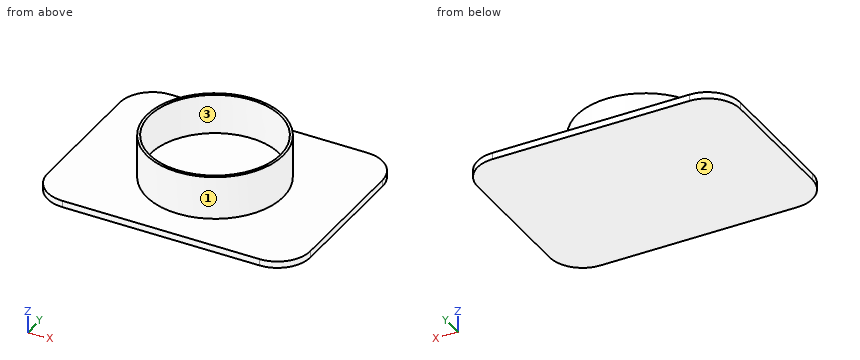
```python
from build123d import *

# Parameters (mm, degrees)
ESQUISSE1_R             = 10.4
BOSS_EXTRU_1_DEPTH      = 6.6
ESQUISSE2_R             = 10
ENL_V_MAT_EXTRU_1_DEPTH = 6
ENL_V_MAT_EXTRU_1_TAPER = 1
ESQUISSE3_W             = 40
ESQUISSE3_H             = 30
BOSS_EXTRU_2_DEPTH      = 1
CONG_1_R                = 5


with BuildPart() as part:
    # Esquisse1 → Boss.-Extru.1 (new body)
    with BuildSketch(Plane.XY):
        Circle(ESQUISSE1_R)
    extrude(amount=BOSS_EXTRU_1_DEPTH)

    # Esquisse2 → Enlèv. mat.-Extru.1 (cut)
    with BuildSketch(Plane.XY.offset(6.6)):
        Circle(ESQUISSE2_R)
    extrude(amount=-ENL_V_MAT_EXTRU_1_DEPTH, taper=ENL_V_MAT_EXTRU_1_TAPER, mode=Mode.SUBTRACT)

    # Esquisse3 → Boss.-Extru.2 (add)
    with BuildSketch(Plane.XY):
        Rectangle(ESQUISSE3_W, ESQUISSE3_H)
    extrude(amount=-BOSS_EXTRU_2_DEPTH)

    # Congé1
    cong_1_edges = [part.edges().sort_by_distance(p)[0] for p in [
        (-20, -15, -0.5),
        (-20, 15, -0.5),
        (20, 15, -0.5),
        (20, -15, -0.5),
    ]]
    fillet(cong_1_edges, radius=CONG_1_R)


solid = part.part
```
Build history of the part. All positions in model axes, mm. Face numbers are marked on the shaded views. Give positions to 0.01 mm unless a question says otherwise; leave off trailing zeros. Loops run counter-clockwise (first coordinate to the right, second up) from the corner with the lowest first, then second, coordinate; pieces in that order, holes last.
Item 1: Flat gauge pins, fed straight in: pin 1 (2 mm diameter, centred on y = -10.5, z = 1.5, fed in from -X); pin 2 (2 mm diameter, centred on x = 8, z = 5.5, fed in from -Y); pin 3 (15 mm diameter, centred on x = 0.5, y = 0.5, fed in from +Z). Where does each tip first touch, or does it go through?
Answers follow:
pin 1: stops at x = -4.23
pin 2: stops at y = -7.69
pin 3: stops at z = 0.6
Item 2: Drill centre lines: line 1 (Z direction, x = -8, y = -10.75); line 2 (Y direction, x = -1, z = 1.25); line 3 (X direction, y = -3, z = 1.75). Where is each one in solid material? Low to high.
Answers follow:
line 1: z = -1 to 0
line 2: y = -10.35 to -9.86, 9.86 to 10.35
line 3: x = -9.96 to -9.45, 9.45 to 9.96
Item 3: Slice it at A-A, the plane z = 4. List the corners of the cut face in (x, y).
Answers follow:
outline: circle Ø20.8 at (0, 0); hole circle Ø19.91 at (0, 0)
Item 4: Pull direction X, two halves, no side cores. Call the marked faces 1, 2 and 3: released by +X, released by -X, zero draft, split by the parting line, or undercut.
Answers follow:
face 1: split by the parting line
face 2: zero draft
face 3: undercut
Item 5: Slice it at B-B, the plane x = 12.5. List the corners of the cut face in (y, z).
Answers follow:
outline: (-15, -1) - (15, -1) - (15, 0) - (-15, 0) - close
Item 6: Slice it at C-C, the plane y = 12. List the corners of the cut face in (x, z), and give its area (3 significant figures).
Answers follow:
outline: (-19.58, -1) - (19.58, -1) - (19.58, 0) - (-19.58, 0) - close
area: 39.2 mm2
